Part model, mm, in its own coordinate system. Round coordinates to 2 decimals unless told otherwise and drop trailing zeros. Write each loop counter-clockwise with the first axis right and the second up, starting at its lowest first coordinate (ties: lowest second). Pieces come first, ordered by that corner, then holes. Notation, with made-up numbers: (23, 19) -> (56, 19) arc R23 cw to (56, 27) -> close; hole circle Ø9 at (56.25, 15). An arc over 180 degrees is marked (long way). Return JSON: item names as keys, results as strings. Group by question number.
(1) Drill centre lines: L1, parallel to X at y = 1.05, z = 0; L2, parallel to Z at x = 50.8, y = 2.15 (3 decimals); L3, parallel to X at y = 2.1, z = 1. Where is each one in solid material? Low to high. Write a range as from..to.
(2) Saw through at A-A (y = 2). List the corners of the cut face in (x, z) (3 decimals).
(3) Drop a flat-ended pin along its axis: pin 1 Ø3 at (x, z) = (-14, 0) entering from -Y. Give the stop position or say it passes through.
(4) Mould opens along Z. For faces 1 (the conical face through (-123.119, 0.145, 18.152)), 2 (the conical face through (123.119, 0.145, -18.152)), 3 (the cylindrical face through (-101.17, 1.54, -1.51)), 4 (the conical face through (114.213, 0.353, 3.258)) say: +Z half, -Z half, draft (parallel to the pull), parting line (faces both ways), or undercut.
(5) Saw through at C-C (x = -50.8). List the corners of the cut face in (y, z) (3 decimals).
(6) Saw through at B-B (x = -107.95). List the corners of the cut face in (y, z) (3 decimals), plus the area to 3 significant figures.
from build123d import *

# Parameters (mm, degrees)
SKETCH1_W                        = 254
SKETCH1_H                        = 44.45
EXTRUDE1_DEPTH                   = 3.048
FILLET1_R                        = 12.7
CHAMFER1_SIZE                    = 0.508
EXTRUDE4_DEPTH                   = 255
F_1_2_CLEARANCE_HOLE4_AT_2_COUNT = 2
F_1_2_CLEARANCE_HOLE4_AT_2_PITCH = 101.6
F_1_2_CLEARANCE_HOLE5_AT_2_COUNT = 2
F_1_2_CLEARANCE_HOLE5_AT_2_PITCH = 215.9


with BuildPart() as part:
    # Sketch1 → Extrude1 (new body)
    with BuildSketch(Plane(origin=(0, 0, 0), x_dir=(1, 0, 0), z_dir=(0, 1, 0))):
        Rectangle(SKETCH1_W, SKETCH1_H)
    extrude(amount=EXTRUDE1_DEPTH)

    # Fillet1
    fillet1_edges = [part.edges().sort_by_distance(p)[0] for p in [
        (-127, 1.524, -22.225),
        (127, 1.524, -22.225),
        (127, 1.524, 22.225),
        (-127, 1.524, 22.225),
    ]]
    fillet(fillet1_edges, radius=FILLET1_R)

    # Chamfer1
    chamfer1_edges = [part.edges().sort_by_distance(p)[0] for p in [
        (0, 0, 22.225),
        (0, 3.048, 22.225),
        (-127, 0, 0),
        (0, 0, -22.225),
        (127, 0, 0),
        (-123.280256121, 0, -18.505256121),
        (123.280256121, 0, -18.505256121),
        (123.280256121, 0, 18.505256121),
        (-123.280256121, 0, 18.505256121),
        (-127, 3.048, 0),
        (127, 3.048, 0),
        (0, 3.048, -22.225),
        (-123.280256121, 3.048, -18.505256121),
        (123.280256121, 3.048, -18.505256121),
        (123.280256121, 3.048, 18.505256121),
        (-123.280256121, 3.048, 18.505256121),
    ]]
    chamfer(chamfer1_edges, length=CHAMFER1_SIZE)

    # Sketch9 → Extrude4 (cut, through all)
    with BuildSketch(Plane(origin=(127, 0, 0), x_dir=(0, 0, -1), z_dir=(1, 0, 0))):
        with BuildLine():
            Line((-1.778, 0), (1.778, 0))
            ThreePointArc((1.778, 0), (0, 0.254), (-1.778, 0))
        make_face()
    extrude(amount=-EXTRUDE4_DEPTH, mode=Mode.SUBTRACT)

    # Sketch10 → 1/2 Clearance Hole4 (revolve, cut)
    with BuildSketch(Plane(origin=(-50.8, 3.048, 0), x_dir=(0, 0, 1), z_dir=(1, 0, 0))):
        Polygon((0, 0), (0, 3.048), (6.985, 3.048), (6.54812, 2.54542705), (6.54812, 0.50257295), (6.985, 0), align=None)
    f_1_2_clearance_hole4 = revolve(axis=Axis((-50.8, 9.398, 0), (0, -1, 0)), mode=Mode.SUBTRACT)

    # 1/2 Clearance Hole4 at 2: 1/2 Clearance Hole4 ×2
    with Locations(*[(i * F_1_2_CLEARANCE_HOLE4_AT_2_PITCH, 0, 0) for i in range(1, F_1_2_CLEARANCE_HOLE4_AT_2_COUNT)]):
        add(f_1_2_clearance_hole4, mode=Mode.SUBTRACT)

    # Sketch12 → 1/2 Clearance Hole5 (revolve, cut)
    with BuildSketch(Plane(origin=(-107.95, 3.048, 0), x_dir=(0, 0, 1), z_dir=(1, 0, 0))):
        Polygon((0, 0), (0, 3.048), (7.366, 3.048), (6.94563, 2.564419633), (6.94563, 0.483580367), (7.366, 0), align=None)
    f_1_2_clearance_hole5 = revolve(axis=Axis((-107.95, 9.398, 0), (0, -1, 0)), mode=Mode.SUBTRACT)

    # 1/2 Clearance Hole5 at 2: 1/2 Clearance Hole5 ×2
    with Locations(*[(i * F_1_2_CLEARANCE_HOLE5_AT_2_PITCH, 0, 0) for i in range(1, F_1_2_CLEARANCE_HOLE5_AT_2_COUNT)]):
        add(f_1_2_clearance_hole5, mode=Mode.SUBTRACT)


solid = part.part
Computed values:
{
 "1": {"L1": "-127..-114.9, -101..-57.35, -44.25..44.25, 57.35..101, 114.9..127", "L2": "-22.225..-6.548, 6.548..22.225", "L3": "-127..-114.82, -101.08..-57.27, -44.33..44.33, 57.27..101.08, 114.82..127"},
 "2": {"outline": "(-127, -9.525) arc R12.7 ccw to (-114.3, -22.225) -> (114.3, -22.225) arc R12.7 ccw to (127, -9.525) -> (127, 9.525) arc R12.7 ccw to (114.3, 22.225) -> (-114.3, 22.225) arc R12.7 ccw to (-127, 9.525) -> close; hole circle Ø13.891 at (-107.95, 0); hole circle Ø13.096 at (-50.8, 0); hole circle Ø13.096 at (50.8, 0); hole circle Ø13.891 at (107.95, 0)"},
 "3": {"pin 1": "y = 0.07"},
 "4": {"face 1": "+Z half", "face 2": "-Z half", "face 3": "undercut", "face 4": "undercut"},
 "5": {"outline": "(0, -21.717) -> (0.508, -22.225) -> (2.54, -22.225) -> (3.048, -21.717) -> (3.048, -6.985) -> (2.545, -6.548) -> (0.503, -6.548) -> (0, -6.985) -> close; (0, 6.985) -> (0.503, 6.548) -> (2.545, 6.548) -> (3.048, 6.985) -> (3.048, 21.717) -> (2.54, 22.225) -> (0.508, 22.225) -> (0, 21.717) -> close"},
 "6": {"outline": "(0, -21.717) -> (0.508, -22.225) -> (2.54, -22.225) -> (3.048, -21.717) -> (3.048, -7.366) -> (2.564, -6.946) -> (0.484, -6.946) -> (0, -7.366) -> close; (0, 7.366) -> (0.484, 6.946) -> (2.564, 6.946) -> (3.048, 7.366) -> (3.048, 21.717) -> (2.54, 22.225) -> (0.508, 22.225) -> (0, 21.717) -> close", "area": "92.2 mm2"}
}
